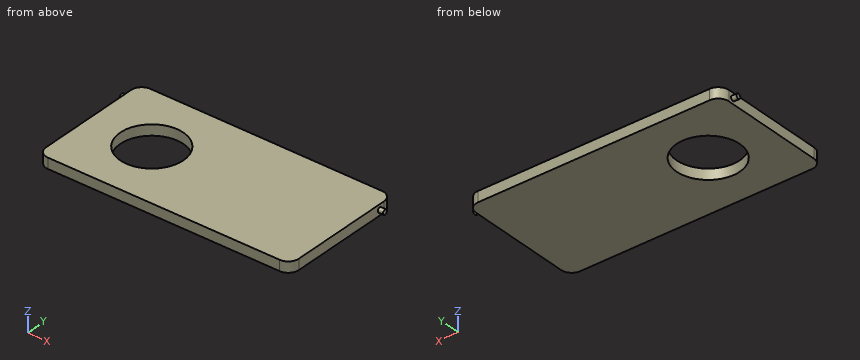
Autodesk Inventor part; units mm, degrees
ref_plane "Plano de trabajo1" through (60, 5, 0) normal (1, 0, 0) x (0, 0, -1)
ref_plane "YZ Plane" through (0, 0, 0) normal (1, 0, 0) x (0, 1, 0)
ref_plane "XZ Plane" through (0, 0, 0) normal (0, 1, 0) x (-1, 0, 0)
sketch "Boceto1" plane through (0, 0, 0) normal (0, 0, 1) x (1, 0, 0)
  line L0 (5, 0) -> (115, 0)
  line L1 (120, 5) -> (120, 55)
  line L2 (115, 60) -> (5, 60)
  line L3 (0, 55) -> (0, 5)
  arc A0 (5, 60) -> (0, 55) centre (5, 55) ccw
  arc A1 (120, 55) -> (115, 60) centre (115, 55) ccw
  arc A2 (115, 0) -> (120, 5) centre (115, 5) ccw
  arc A3 (0, 5) -> (5, 0) centre (5, 5) ccw
  point P0 (0, 0)
  point P1 (120, 60)
  point P2 (120, 0)
  point P3 (0, 60)
  dimension "d0" = 120
  dimension "d1" = 60
  dimension "d2" = 5
extrude "Extrusión1" add sketch "Boceto1" along normal blind 5
sketch "Boceto2" plane through (120, 5, 0) normal (1, 0, 0) x (0, 0, -1)
  point P0 (0, -5)
sketch "Boceto3" plane through (120, 5, 0) normal (1, 0, 0) x (0, 0, -1)
  circle A0 centre (-2.5, 47.5) radius 1.15
  line L0 (-5, 0) -> (-5, 50)
  line L1 (0, 50) -> (-5, 50)
  point P0 (0, -5)
  dimension "d5" = 2.3
  dimension "d6" = 2.5
  dimension "d7" = 2.5
extrude "Extrusión2" add sketch "Boceto3" along normal blind 2.5
ref_plane "Plano de trabajo1" through (60, 5, 0) normal (1, 0, 0) x (0, 0, -1)
mirror "Simetría1" about plane through (60, 5, 0) normal (1, 0, 0) of "Extrusión2"
sketch "Boceto4" plane through (0, 0, 5) normal (0, 0, 1) x (1, 0, 0)
  circle A0 centre (30, 30) radius 15
  line L0 (0, 55) -> (0, 5)
  point P0 (0, 0)
  point P1 (0, 30)
  dimension "d10" = 30
  dimension "d11" = 30
extrude "Extrusión3" cut sketch "Boceto4" against normal through all
properties part number "Puerta" material "Plástico ABS"
CAD build for the part. Positions are in the model's coordinates, mm. Round coordinates to 2 decimals unless told otherwise and drop trailing zeros. Loops run counter-clockwise (first coordinate to the right, second up) from the corner with the lowest first, then second, coordinate; pieces in that order, holes last. Notation, with made-up numbers: M -10.5,57.5 L -4.5,57.5 A20 ccw -4.5,73.5 Z; hole C 36.25,-6.5 d6. An arc over 180 degrees is marked long. Return JSON: item names as keys, results as strings. Group by question number.
(1) Saw through at A-A, the plane y = 30. List the corners of the cut face in (x, z).
(2) Saw through at B-B, the plane z = 2.5. List the corners of the cut face in (x, y).
(3) Wall check: probe 1 along Y at (x, z) = (30, 2.1); probe 2 along X at (y, z) = (13, 2.65); probe 3 along X at (y, z) = (26, 4.7). Give the ranges that are in metal, low to high. Write a range as [from, to].
(4) Saw through at C-C, the plane x = 30. List the corners of the cut face in (y, z).
(5) Saw through at D-D, the plane y = 52.5. List the corners of the cut face in (x, z).
(6) Drop a flat-ended pin along its axis: P1, Ø1, axis at y = 37.5, z = 4.5, coming from the +X side. Give the stop position or say it passes through.
Answer list:
{
 "1": {"outline": "M 0,0 L 15,0 L 15,5 L 0,5 Z; M 45,0 L 120,0 L 120,5 L 45,5 Z"},
 "2": {"outline": "M -2.5,51.35 L 0,51.35 L 0,5 A5 ccw 5,0 L 115,0 A5 ccw 120,5 L 120,51.35 L 122.5,51.35 L 122.5,53.65 L 120,53.65 L 120,55 A5 ccw 115,60 L 5,60 A5 ccw 0,55 L 0,53.65 L -2.5,53.65 Z; hole C 30,30 d30"},
 "3": {"probe 1": "[0, 15], [45, 60]", "probe 2": "[0, 120]", "probe 3": "[0, 15.54], [44.46, 120]"},
 "4": {"outline": "M 0,0 L 15,0 L 15,5 L 0,5 Z; M 45,0 L 60,0 L 60,5 L 45,5 Z"},
 "5": {"outline": "M -2.5,1.35 L 0,1.35 L 0,0 L 120,0 L 120,1.35 L 122.5,1.35 L 122.5,3.65 L 120,3.65 L 120,5 L 0,5 L 0,3.65 L -2.5,3.65 Z"},
 "6": {"P1": "x = 120"}
}
